Job drawing, mm, ordinate dimensions from the low corner. One solid piece. Round coordinates to 2 decimals unless told otherwise and drop trailing zeros. Order: outer loops, then holes, each group sorted by start corner. A loop starts at its lowest first (then second) coordinate and runs counter-clockwise, first axis right, second up. Notation, with made-up numbers: (-7, 32.5) -> (15, 32.5) arc R31 cw to (15, 56.5) -> close; hole circle Ø5 at (19.25, 38). An arc over 180 degrees is marked (long way). Return JSON: item names as keys, results as strings. Group by question number.
Q1. Probe line 1 along X through (y, z) = (18, 76) (1 decimal); line 2 along Z through (x, y) = (196.5, 38.5); line 3 along X through (y, z) = (26, 59.5) (1 decimal). List the from-to ranges inside material, lowest first.
Q2. Cut at C-C (x = 133.35). Write the cut outline in (y, z).
Q3. Flat gauge pin, fed straight in: pin 1 (8 mm diameter, centred on x = 231.5, z = 38.5, fed in from -Y). Where does the tip first touch, or does it go through?
Q4. Cut at A-A (z = 76.2). Count the separate pieces of the cut face and the enclosed holes in it, then the cut area to 3 significant figures.
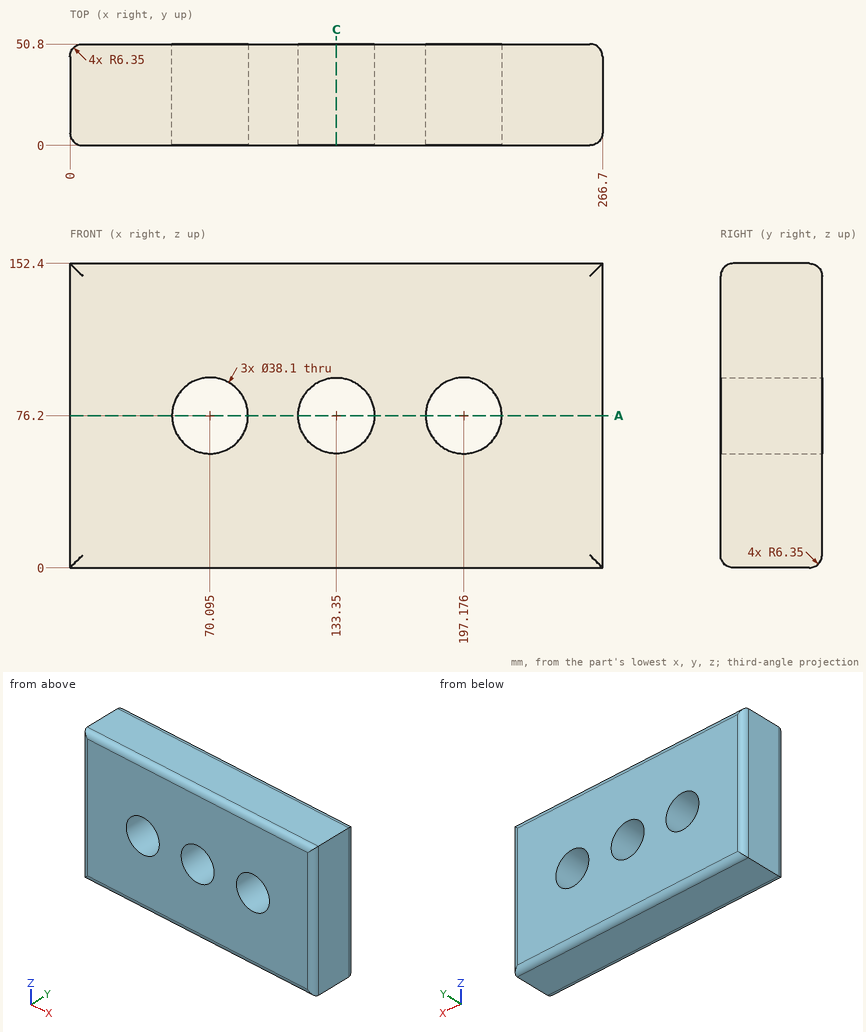
Solution:
{
 "1": {"line 1": "x = 0 to 51, 89.1 to 114.3, 152.4 to 178.1, 216.2 to 266.7", "line 2": "z = 0 to 57.16, 95.24 to 152.4", "line 3": "x = 0 to 60.9, 79.3 to 124.2, 142.5 to 188, 206.3 to 266.7"},
 "2": {"outline": "(0, 6.35) arc R6.35 ccw to (6.35, 0) -> (44.45, 0) arc R6.35 ccw to (50.8, 6.35) -> (50.8, 57.15) -> (0, 57.15) -> close; (0, 95.25) -> (50.8, 95.25) -> (50.8, 146.05) arc R6.35 ccw to (44.45, 152.4) -> (6.35, 152.4) arc R6.35 ccw to (0, 146.05) -> close"},
 "3": {"pin 1": "stops at y = 0"},
 "4": {"separate pieces": "4", "enclosed holes": "0", "area": "7,710 mm²"}
}
